Part model, mm, in its own coordinate system. A direction names the side the tool comes from. Coordinates: 2 decimals unless noted, no trailing zeros. Write each loop counter-clockwise with the first axis right and the second up, starting at its lowest first coordinate (ties: lowest second). Pieces come first, ordered by that corner, then holes. Notation, with made-up numbers: (25, 22.5) - (78, 22.5) arc R12 cw to (78, 28.5) - close; hole circle Ø7 at (-10, 77). An arc over 180 degrees is marked (long way). Use a Markdown table: item, result.
```python
from build123d import *


with BuildPart() as f2:
    # F2: sweep along a path in F0
    with BuildLine(Plane.XZ) as f2_path:
        Line((0, 0), (0, 51.4572679996))
        ThreePointArc((0, 51.4572679996), (-29.1573684376, 121.8493823248), (-99.5494827628, 151.0067507625))
        Line((-99.5494827628, 151.0067507625), (-208.2385346019, 151.0067507625))
    # F1 (on Top) → F2 (sweep)
    with BuildSketch(Plane.XY):
        with BuildLine():
            ThreePointArc((-17.9969767891, -41.5336991378), (-14.094527486, -41.9556359374), (-10.6398630821, -40.0921888406))
            ThreePointArc((-10.6398630821, -40.0921888406), (5.7210400439, 0.2988613285), (-11.0602959901, 40.517051812))
            ThreePointArc((-11.0602959901, 40.517051812), (-14.0530889357, 42.1143611499), (-17.428490612, 41.7754359954))
            ThreePointArc((-17.428490612, 41.7754359954), (-45.2641572804, 0.3088742632), (-17.9969767891, -41.5336991378))
        make_face()
    sweep(path=f2_path.line)


solid = f2.part
```
Item 1: Drill centre lines: probe 1 along Z at (x, y) = (-135, 2); probe 2 along X at (y, z) = (4, 28); probe 3 along Z at (x, y) = (-126, -28). Where is each one in solid material? Low to high.
From the geometry:
| item | result |
|---|---|
| probe 1 | 105.79 to 156.69 |
| probe 2 | -45.09 to 5.58 |
| probe 3 | 115.44 to 149.42 |
Item 2: Which spindle directions (+Z, -Z, +X, -X, +Y, -Y) get a long thin tool onto all of the face, cutting with end or side? Do faces 1 (the face through (-154.655, -41.966, 136.857)), 2 (the face through (-14.149, -41.966, 26.089)), 3 (the face through (-154.655, 42.105, 137.001)), 4 (the face through (-154.655, 1.049, 105.754)). Say none if no direction does.
From the geometry:
| item | result |
|---|---|
| face 1 | -X, -Y |
| face 2 | -Z, -Y |
| face 3 | -X, +Y |
| face 4 | -Z, -X |
Item 3: Drop flat-ended pins along their axis: P1, Ø6, axis at x = -88.5, y = -5, coming from the +Z side; P2, Ø12, axis at x = -60.5, y = -19, coming from the -Z side; P3, Ø6, axis at x = -96, y = 30, coming from the +Z side. Give the stop position or say it passes through.
From the geometry:
| item | result |
|---|---|
| P1 | z = 156.28 |
| P2 | z = 87.7 |
| P3 | z = 149.91 |
Item 4: Band-saw the part on A-A, the plane x = -131.5. Give the cut face in (y, z).
From the geometry:
| item | result |
|---|---|
| outline | (-41.53, 133.01) arc R45.27 ccw to (41.78, 133.58) arc R5.83 ccw to (40.52, 139.95) arc R57.3 ccw to (-40.09, 140.37) arc R6.62 ccw to start |
Item 5: Band-saw the part on B-B, the plane z = 14.5. Give the cut face in (x, y), then the cut area to 3 significant figures.
From the geometry:
| item | result |
|---|---|
| outline | (-18, -41.53) arc R6.62 ccw to (-10.64, -40.09) arc R57.3 ccw to (-11.06, 40.52) arc R5.83 ccw to (-17.43, 41.78) arc R45.27 ccw to start |
| area | 3,150 mm^2 |
